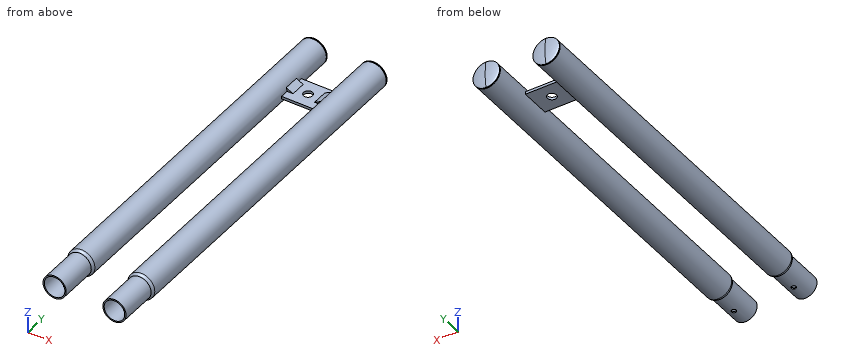
from build123d import *
from build123d.topology import SkipClean

# Parameters (mm, degrees)
SKETCH1_W                = 28
SKETCH1_H                = 25
SKETCH1_R                = 3.8
BOSS_EXTRUDE1_DEPTH      = 1.1
BOSS_EXTRUDE2_DEPTH      = 241
BOSS_EXTRUDE2_DEPTH_BACK = 57
SKETCH2_R                = 11.15
SKETCH2_R_2              = 10.05
SKETCH3_R                = 11.15
SKETCH3_R_2              = 8.65
BOSS_EXTRUDE3_DEPTH      = 1.1
SKETCH4_R                = 9.75
SKETCH4_R_2              = 8.65
BOSS_EXTRUDE4_DEPTH      = 32
FILLET1_R                = 3
CUT_EXTRUDE1_REACH       = 290.014
CUT_EXTRUDE1_END_RADIUS  = 9.75
SKETCH8_R                = 2
CHAMFER1_SIZE            = 0.3
BOSS_EXTRUDE5_DEPTH      = 25
BOSS_EXTRUDE5_2_DEPTH    = 25
BOSS_EXTRUDE6_START      = -5
BOSS_EXTRUDE6_DEPTH      = 13


with BuildPart() as part:
    # Sketch1 → Boss-Extrude1 (new, symmetric)
    with BuildSketch(Plane.XY):
        Rectangle(SKETCH1_W, SKETCH1_H)
        Circle(SKETCH1_R, mode=Mode.SUBTRACT)
    extrude(amount=BOSS_EXTRUDE1_DEPTH, both=True)


with BuildPart() as body_2:
    # Sketch2 → Boss-Extrude2 (new, two sides: drawn at the far end of the back side and taken through both)
    with BuildSketch(Plane.XZ.offset(12.5).offset(-BOSS_EXTRUDE2_DEPTH_BACK)):
        with Locations(Location((-25.15, 0, 0), (0, 0, 270))):
            Circle(SKETCH2_R)
        with Locations(Location((-25.15, 0, 0), (0, 0, 270))):
            Circle(SKETCH2_R_2, mode=Mode.SUBTRACT)
    extrude(amount=BOSS_EXTRUDE2_DEPTH + BOSS_EXTRUDE2_DEPTH_BACK)

    # Sketch3 → Boss-Extrude3 (add)
    with BuildSketch(Plane.XZ.offset(253.5)):
        with Locations(Location((-25.15, 0, 0), (0, 0, 270))):
            Circle(SKETCH3_R)
        with Locations(Location((-25.15, 0, 0), (0, 0, 270))):
            Circle(SKETCH3_R_2, mode=Mode.SUBTRACT)
    extrude(amount=-BOSS_EXTRUDE3_DEPTH)

    # Sketch4 → Boss-Extrude4 (add)
    with SkipClean():  # the faces are left unmerged after this step: merging them gives an invalid solid
        with BuildSketch(Plane.XZ.offset(253.5)):
            with Locations(Location((-25.15, 0, 0), (0, 0, 270))):
                Circle(SKETCH4_R)
            with Locations(Location((-25.15, 0, 0), (0, 0, 270))):
                Circle(SKETCH4_R_2, mode=Mode.SUBTRACT)
        extrude(amount=BOSS_EXTRUDE4_DEPTH)

    # Fillet1
    # the kernel refuses this fillet: 3 mm, written as the material it adds along each edge
    with BuildSketch(Plane(origin=(-25.15, -252.4, 0), x_dir=(0, 0, -1), z_dir=(1, 0, 0))) as fillet1_piece_1:
        with BuildLine():
            CenterArc((7.05, 2.537715508), FILLET1_R, 302.230952635, 57.769047365)
            Line((8.65, 0), (8.682, -0.05075431))
            ThreePointArc((8.682, -0.05075431), (9.35, -0.06), (10.05, -0.06))
            Line((10.05, -0.06), (10.11, 0))
            Line((10.11, 0), (10.11, 2.537715508))
            Line((10.11, 2.537715508), (10.05, 2.537715508))
        make_face()
    revolve(axis=Axis((-25.15, -252.4, 0), (0, 1, 0)))
    # the kernel refuses this fillet: 3 mm, written as the material it takes off along each edge
    with BuildSketch(Plane(origin=(-25.15, -253.5, 0), x_dir=(0, 0, -1), z_dir=(-1, 0, 0))) as fillet1_2_piece_1:
        with BuildLine():
            CenterArc((8.15, -2.537715508), FILLET1_R, 0, 57.769047365)
            Line((9.75, 0), (9.782, 0.05075431))
            ThreePointArc((9.782, 0.05075431), (10.45, 0.06), (11.15, 0.06))
            Line((11.15, 0.06), (11.21, 0))
            Line((11.21, 0), (11.21, -2.537715508))
            Line((11.21, -2.537715508), (11.15, -2.537715508))
        make_face()
    revolve(axis=Axis((-25.15, -253.5, 0), (0, -1, 0)), mode=Mode.SUBTRACT)

    # Cut-Extrude1: up to this cylinder (the profile starts inside it)
    cut_extrude1_end = Plane(origin=(-25.15, -270.5, 0), z_dir=(0, 1, 0)) * Cylinder(CUT_EXTRUDE1_END_RADIUS, 600.528, mode=Mode.PRIVATE)
    # Sketch8 → Cut-Extrude1 (cut, up to the surface)
    with BuildSketch(Plane.XY, mode=Mode.PRIVATE) as cut_extrude1_sk1:
        with Locations((-25.15, -270.5)):
            Circle(SKETCH8_R)
    cut_extrude1_tool1 = extrude(cut_extrude1_sk1.sketch, amount=-CUT_EXTRUDE1_REACH, mode=Mode.PRIVATE) & cut_extrude1_end
    add(cut_extrude1_tool1.solids().sort_by_distance((-25.15, -270.5, 0))[0], mode=Mode.SUBTRACT)


with BuildPart() as body_3:
    # Sketch5 → Revolve1 (revolve)
    with SkipClean():  # the faces are left unmerged after this step: merging them gives an invalid solid
        with BuildSketch(Plane.XY, mode=Mode.PRIVATE) as revolve1_sk:
            with BuildLine():
                add(Edge.make_bspline(
                    [(-14, 45.5), (-14, 47), (-25.15, 47)],
                    knots=[3.141592654, 3.141592654, 3.141592654, 4.71238898, 4.71238898, 4.71238898], degree=2, weights=[1, 0.707106781, 1]))
                Line((-25.15, 47), (-25.15, 45.5))
                Line((-25.15, 45.5), (-14, 45.5))
            make_face()
            with BuildLine():
                Line((-25.15, 45.5), (-25.15, 47))
                add(Edge.make_bspline(
                    [(-25.15, 47), (-36.3, 47), (-36.3, 45.5)],
                    knots=[4.71238898, 4.71238898, 4.71238898, 6.283185307, 6.283185307, 6.283185307], degree=2, weights=[1, 0.707106781, 1]))
                Line((-36.3, 45.5), (-25.15, 45.5))
            make_face()
            with BuildLine():
                Line((-14, 45.5), (-25.15, 45.5))
                Line((-25.15, 45.5), (-25.15, 44.5))
                Line((-25.15, 44.5), (-16.839280684, 44.5))
                add(Edge.make_bspline(
                    [(-16.839280684, 44.5), (-14, 44.927050983), (-14, 45.5)],
                    knots=[2.411864997, 2.411864997, 2.411864997, 3.141592654, 3.141592654, 3.141592654], degree=2, weights=[1, 0.934172359, 1]))
            make_face()
            with BuildLine():
                Line((-25.15, 44.5), (-25.15, 45.5))
                Line((-25.15, 45.5), (-36.3, 45.5))
                add(Edge.make_bspline(
                    [(-36.3, 45.5), (-36.3, 44.927050983), (-33.460719316, 44.5)],
                    knots=[0, 0, 0, 0.729727656, 0.729727656, 0.729727656], degree=2, weights=[1, 0.934172359, 1]))
                Line((-33.460719316, 44.5), (-25.15, 44.5))
            make_face()
            with BuildLine():
                add(Edge.make_bspline(
                    [(-36.3, 45.5), (-36.3, 44.927050983), (-33.460719316, 44.5)],
                    knots=[0, 0, 0, 0.729727656, 0.729727656, 0.729727656], degree=2, weights=[1, 0.934172359, 1]))
                Line((-36.3, 45.5), (-36.3, 44.5))
                Line((-36.3, 44.5), (-33.460719316, 44.5))
            make_face()
        revolve(revolve1_sk.sketch.rotate(Axis((-25.15, 47, 0), (0, -1, 0)), 270), axis=Axis((-25.15, 47, 0), (0, -1, 0)))
    add(body_3.part.scale(1), mode=Mode.REPLACE)  # the faces are merged on a copy

    # Chamfer1
    chamfer1_edges = [body_3.edges().sort_by_distance(p)[0] for p in [
        (-25.15, 44.5, -11.15),
    ]]
    chamfer(chamfer1_edges, length=CHAMFER1_SIZE)


with BuildPart() as body_4:
    # Sketch6 → Boss-Extrude5 (new body)
    with BuildSketch(Plane(origin=(0, 12.5, 0), x_dir=(1, 0, 0), z_dir=(0, 1, 0))):
        with BuildLine():
            Line((-14, 0), (-14, 1.1))
            Line((-14, 1.1), (-14.054392761, 1.1))
            ThreePointArc((-14.054392761, 1.1), (-14.013606492, 0.550671992), (-14, 0))
        make_face()
    extrude(amount=-BOSS_EXTRUDE5_DEPTH)


with BuildPart() as body_5:
    # Sketch6 → Boss-Extrude5 2 (new body)
    with BuildSketch(Plane(origin=(0, 12.5, 0), x_dir=(1, 0, 0), z_dir=(0, 1, 0))):
        with BuildLine():
            Line((-14, -1.1), (-14, 0))
            ThreePointArc((-14, 0), (-14.013606492, -0.550671992), (-14.054392761, -1.1))
            Line((-14.054392761, -1.1), (-14, -1.1))
        make_face()
    extrude(amount=-BOSS_EXTRUDE5_2_DEPTH)


with BuildPart() as body_6:
    # Sketch7 → Boss-Extrude6 (new body)
    with BuildSketch(Plane(origin=(0, 12.5, 0), x_dir=(1, 0, 0), z_dir=(0, 1, 0)).offset(BOSS_EXTRUDE6_START)):
        with BuildLine():
            Line((-14.781176537, -4.1), (-9.054392761, -1.1))
            Line((-9.054392761, -1.1), (-14, -1.1))
            Line((-14, -1.1), (-14.054392761, -1.1))
            ThreePointArc((-14.054392761, -1.1), (-14.313467052, -2.625272112), (-14.781176537, -4.1))
        make_face()
    extrude(amount=-BOSS_EXTRUDE6_DEPTH)


with BuildPart() as body_7:
    # Mirror1: mirrored copy
    add(body_2.part.mirror(Plane(origin=(0, 0, 0), x_dir=(0, 0, 1), z_dir=(1, 0, 0))))


with BuildPart() as body_8:
    # Mirror1 2: mirrored copy
    add(body_3.part.mirror(Plane(origin=(0, 0, 0), x_dir=(0, 0, 1), z_dir=(1, 0, 0))))


with BuildPart() as body_9:
    # Mirror1 3: mirrored copy
    add(body_4.part.mirror(Plane(origin=(0, 0, 0), x_dir=(0, 0, 1), z_dir=(1, 0, 0))))


with BuildPart() as body_10:
    # Mirror1 4: mirrored copy
    add(body_5.part.mirror(Plane(origin=(0, 0, 0), x_dir=(0, 0, 1), z_dir=(1, 0, 0))))


with BuildPart() as body_11:
    # Mirror1 5: mirrored copy
    add(body_6.part.mirror(Plane(origin=(0, 0, 0), x_dir=(0, 0, 1), z_dir=(1, 0, 0))))


with BuildPart() as part_1:
    add(part.part)

    # Combine1: union body 2, body 3, body 4, body 5, body 6, body 7, body 8, body 9, body 10, body 11
    add(body_2.part)
    add(body_3.part)
    add(body_4.part)
    add(body_5.part)
    add(body_6.part)
    add(body_7.part)
    add(body_8.part)
    add(body_9.part)
    add(body_10.part)
    add(body_11.part)


solid = part_1.part
For this review, take the finished solid that the model builds, in its own axes (mm). Round coordinates to 2 decimals unless told otherwise and drop trailing zeros. Order: outer loops, then holes, each group sorted by start corner. A loop starts at its lowest first (then second) coordinate and runs counter-clockwise, first axis right, second up. Notation, with made-up numbers: M -28,3 L 13,3 A23 cw 13,19 Z; hole C 83,18.5 d4. An arc over 180 degrees is marked long. Use a Markdown table: item, result. Add a question column.
Item 1: Add section A-A, the plane y = 0. Give the boundary of the cut face in (x, z).
Item 2: Add section B-B, the plane x = 0. Give the boundary of the cut face in (y, z), then the cut area to 3 significant figures.
Item 3: Add section C-C, the plane y = -63. Give the boundary of the cut face in (x, z), then the cut area to 3 significant figures.
Item 4: Insertion check: pin 1 (3.5 mm diameter, centred on x = 11.5, z = 3, fed in from -Y); pin 2 (7 mm diameter, centred on x = 0, y = 0, fed in from -Z); pin 3 (5 mm diameter, centred on x = -15.5, z = -2.5, fed in from +Y); pin 4 (8 mm diameter, centred on y = -126.5, z = -6, fed in from -X). Each pin has a flat end and moves straight along its axis. Give the tip position at first contact, or say it passes through.
Item 5: To check wall thickness, follow line 1 along X through (y, z) = (-276, 0); line 2 along X through (y, z) = (-60.5, 0); line 3 along Z through (x, y) = (26, -149). State the ranges of each line that lie inside material, in increasing order.
Geometry results:
| question | item | result |
|---|---|---|
| 1 | outline | M -14.78,4.1 A11.15 ccw long -14.05,-1.1 L -3.8,-1.1 L -3.8,1.1 L -9.05,1.1 Z; M 3.8,-1.1 L 14.05,-1.1 A11.15 ccw long 14.78,4.1 L 9.05,1.1 L 3.8,1.1 Z; hole C -25.15,0 d20.1; hole C 25.15,0 d20.1 |
| 2 | outline | M -12.5,-1.1 L -3.8,-1.1 L -3.8,1.1 L -12.5,1.1 Z; M 3.8,-1.1 L 12.5,-1.1 L 12.5,1.1 L 3.8,1.1 Z |
| 2 | area | 38.3 mm² |
| 3 | outline | C -25.15,0 d22.3; C 25.15,0 d22.3; hole C -25.15,0 d20.1; hole C 25.15,0 d20.1 |
| 3 | area | 147 mm² |
| 4 | pin 1 | stops at y = -5.5 |
| 4 | pin 2 | passes through |
| 4 | pin 3 | stops at y = 46.61 |
| 4 | pin 4 | stops at x = -36.12 |
| 5 | line 1 | x = -34.9 to -33.8, -16.5 to -15.4, 15.4 to 16.5, 33.8 to 34.9 |
| 5 | line 2 | x = -36.3 to -35.2, -15.1 to -14, 14 to 15.1, 35.2 to 36.3 |
| 5 | line 3 | z = -11.12 to -10.01, 10.01 to 11.12 |
